from build123d import *

# Parameters (mm, degrees)
SKETCH_1_R               = 2
SKETCH_1_R_2             = 10
EXTRUDE_1_DEPTH          = 20
SKETCH_2_R               = 25
SKETCH_2_R_2             = 12
EXTRUDE_2_DEPTH          = 2
EXTRUDE_3_DEPTH          = 110
SKETCH_4_OUTSIDE_W       = 274.729
SKETCH_4_OUTSIDE_H       = 190.272
CUT_EXTRUDE_5_DEPTH      = 62
CUT_EXTRUDE_5_DEPTH_BACK = 62
SKETCH_5_R               = 7.5
EXTRUDE_4_DEPTH          = 55
SKETCH_6_R               = 5
EXTRUDE_5_DEPTH          = 40


with BuildPart() as part:
    # Эскиз1 → Бобышка-Вытянуть1 (new body)
    with BuildSketch(Plane(origin=(0, 0, 0), x_dir=(1, 0, 0), z_dir=(0, 1, 0))):
        with BuildLine():
            Line((35, 12.5), (35, -37))
            ThreePointArc((35, -37), (28.263455967, -53.263455967), (12, -60))
            Line((12, -60), (11, -60))
            Line((11, -60), (11, -67))
            ThreePointArc((11, -67), (10.121320344, -69.121320344), (8, -70))
            Line((8, -70), (-8, -70))
            ThreePointArc((-8, -70), (-10.121320344, -69.121320344), (-11, -67))
            Line((-11, -67), (-11, -60))
            Line((-11, -60), (-12, -60))
            ThreePointArc((-12, -60), (-28.263455967, -53.263455967), (-35, -37))
            Line((-35, -37), (-35, -35))
            Line((-35, -35), (-37, -35))
            ThreePointArc((-37, -35), (-39.121320344, -34.121320344), (-40, -32))
            Line((-40, -32), (-40, 12.5))
            ThreePointArc((-40, 12.5), (-40.878679656, 14.621320344), (-43, 15.5))
            Line((-43, 15.5), (-49, 15.5))
            ThreePointArc((-49, 15.5), (-57.485281374, 19.014718626), (-61, 27.5))
            Line((-61, 27.5), (-61, 28))
            ThreePointArc((-61, 28), (-57.485281374, 36.485281374), (-49, 40))
            Line((-49, 40), (49, 40))
            ThreePointArc((49, 40), (57.485281374, 36.485281374), (61, 28))
            Line((61, 28), (61, 27.5))
            ThreePointArc((61, 27.5), (57.485281374, 19.014718626), (49, 15.5))
            Line((49, 15.5), (38, 15.5))
            ThreePointArc((38, 15.5), (35.878679656, 14.621320344), (35, 12.5))
        make_face()
        with Locations((27.5, 27.5)):
            Circle(SKETCH_1_R, mode=Mode.SUBTRACT)
        with Locations((-27.5, 27.5)):
            Circle(SKETCH_1_R, mode=Mode.SUBTRACT)
        with Locations((-27.5, -27.5)):
            Circle(SKETCH_1_R, mode=Mode.SUBTRACT)
        with Locations((27.5, -27.5)):
            Circle(SKETCH_1_R, mode=Mode.SUBTRACT)
        Circle(SKETCH_1_R_2, mode=Mode.SUBTRACT)
    extrude(amount=EXTRUDE_1_DEPTH)

    # Эскиз2 → Бобышка-Вытянуть2 (add)
    with BuildSketch(Plane.XZ):
        Circle(SKETCH_2_R)
        Circle(SKETCH_2_R_2, mode=Mode.SUBTRACT)
    extrude(amount=EXTRUDE_2_DEPTH)

    # Эскиз3 → Бобышка-Вытянуть3 (add)
    with BuildSketch(Plane(origin=(0, 20, 0), x_dir=(1, 0, 0), z_dir=(0, 1, 0))):
        with BuildLine():
            Line((-37.583733624, -32.103535028), (-37.583733624, 36.457416544))
            Line((-37.583733624, 36.457416544), (-16, 36.457416544))
            Line((-16, 36.457416544), (-16, 146.457416544))
            Line((-16, 146.457416544), (16, 146.457416544))
            Line((16, 146.457416544), (16, 36.457416544))
            Line((16, 36.457416544), (33.766635678, 36.457416544))
            Line((33.766635678, 36.457416544), (33.766635678, -32.103535028))
            ThreePointArc((33.766635678, -32.103535028), (28.080470389, -50.220903637), (11.304482379, -59.11684357))
            Line((11.304482379, -59.11684357), (-11, -59.11684357))
            ThreePointArc((-11, -59.11684357), (-27.23731375, -51.101673534), (-33.326201299, -34.048264581))
            Line((-33.326201299, -34.048264581), (-37.583733624, -32.103535028))
        make_face()
    extrude(amount=EXTRUDE_3_DEPTH)

    # Эскиз4 outside → Вырез-Вытянуть5 (cut, two sides)
    with BuildSketch(Plane(origin=(0, 0, 0), x_dir=(0, 0, -1), z_dir=(1, 0, 0))) as cut_extrude_5_sk:
        with Locations((38.2285, 64)):
            Rectangle(SKETCH_4_OUTSIDE_W, SKETCH_4_OUTSIDE_H)
        Polygon((-59.11684357, 111.009140669), (-59.11684357, 20), (-70, 20), (-70, 0), (-25.61704501, 0), (-25.61704501, -2.465693048), (25.5, -2.465693048), (25.5, 0), (40, 0), (40, 20), (36.457416544, 20), (36.457416544, 70.826498743), (84.412407161, 70.826498743), (128.193178806, 61.67378586), (131.933723793, 56.499947934), (146.457416544, 56.499947934), (146.457416544, 83.32776512), (75.121913518, 98.241010205), (43.39244845, 98.241010205), (36.457416544, 102.079664685), (36.457416544, 126.416047598), (31.26241492, 130), (-26.036858243, 130), align=None, mode=Mode.SUBTRACT)
    extrude(amount=CUT_EXTRUDE_5_DEPTH, mode=Mode.SUBTRACT)
    extrude(cut_extrude_5_sk.sketch, amount=-CUT_EXTRUDE_5_DEPTH_BACK, mode=Mode.SUBTRACT)

    # Эскиз5 → Бобышка-Вытянуть4 (add)
    with BuildSketch(Plane.XZ.offset(-20)):
        Circle(SKETCH_5_R)
    extrude(amount=EXTRUDE_4_DEPTH)

    # Эскиз6 → Бобышка-Вытянуть5 (add)
    with BuildSketch(Plane.XZ.offset(35)):
        Circle(SKETCH_6_R)
    extrude(amount=EXTRUDE_5_DEPTH)


solid = part.part
CAD build for the part. Positions are in the model's coordinates, mm. A direction names the side the tool comes from. Coordinates: 2 decimals unless noted, no trailing zeros. Order: outer loops, then holes, each group sorted by start corner. A loop starts at its lowest first (then second) coordinate and runs counter-clockwise, first axis right, second up. Notation, with made-up numbers: (59.25, 52.25) -> (94.25, 52.25) arc R19 ccw to (94.25, 70.25) -> close; hole circle Ø10 at (50, 70.5). An arc over 180 degrees is marked (long way). Answer in a Markdown table with one row per item.
1) Drill centre lines: line 1 (Z direction, x = 0, y = 10.5); line 2 (Z direction, x = 27.5, y = 10.5); line 3 (Y direction, x = 52.5, z = -33). Where is each one in solid material? Low to high.
Check values:
| item | result |
|---|---|
| line 1 | -40 to -10, -7.5 to 7.5, 10 to 70 |
| line 2 | -40 to -29.5, -25.5 to 25.5, 29.5 to 53.99 |
| line 3 | 0 to 20 |
2) Mould opens along X. For faces 5 (the face through (-27.063, 71.963, 51.295)), 6 (the face through (0, 98.241, -59)), 7 (the face through (-2.17, 9.86, 9.76)) say: pulls with the +X half, pulls with the -X half, needs draft (parallel to the pull), parting line crosses it, or undercut.
Check values:
| item | result |
|---|---|
| face 5 | pulls with the -X half |
| face 6 | needs draft |
| face 7 | undercut |
3) Band-saw the part on A-A (y = 44). List the corners of the cut face in (x, z).
Check values:
| item | result |
|---|---|
| outline | (-37.58, -36.46) -> (33.77, -36.46) -> (33.77, 32.1) arc R25 ccw to (11.3, 59.12) -> (-11, 59.12) arc R24.13 ccw to (-33.33, 34.05) -> (-37.58, 32.1) -> close |
4) Band-saw the part on D-D (z = 22). List the corners of the cut face in (x, y), and give its area (3 significant figures).
Check values:
| item | result |
|---|---|
| outline | (-40, 0) -> (-11.87, 0) -> (-11.87, -2) -> (11.87, -2) -> (11.87, 0) -> (35, 0) -> (35, 20) -> (33.77, 20) -> (33.77, 130) -> (-37.58, 130) -> (-37.58, 20) -> (-40, 20) -> close |
| area | 9,400 mm2 |
5) Flat gauge pins, fed straight in: P1, Ø3, axis at x = 27.5, z = -27.5, coming from the -Y side; P2, Ø6, axis at y = 5.5, z = 11, coming from the +X side; P3, Ø0.8, axis at x = -11.5, y = 9.5, coming from the +Z side; P4, Ø4.5, axis at x = 27.5, z = 27.5, coming from the +Y side. Where does each tip first touch, or does it go through?
Check values:
| item | result |
|---|---|
| P1 | y = 20 |
| P2 | x = 35 |
| P3 | z = 60 |
| P4 | y = 130 |
6) Band-saw the part on C-C (y = 115.5). List the corners of the cut face in (x, z).
Check values:
| item | result |
|---|---|
| outline | (-37.58, -36.46) -> (33.77, -36.46) -> (33.77, 32.1) arc R25 ccw to (27.13, 51.29) -> (-27.06, 51.29) arc R24.13 ccw to (-33.33, 34.05) -> (-37.58, 32.1) -> close |
7) Band-saw the part on B-B (z = 0). List the corners of the cut face in (x, y).
Check values:
| item | result |
|---|---|
| outline | (-40, 0) -> (-25, 0) -> (-25, -2) -> (-12, -2) -> (-12, 0) -> (-10, 0) -> (-10, 20) -> (-7.5, 20) -> (-7.5, -35) -> (-5, -35) -> (-5, -75) -> (5, -75) -> (5, -35) -> (7.5, -35) -> (7.5, 20) -> (10, 20) -> (10, 0) -> (12, 0) -> (12, -2) -> (25, -2) -> (25, 0) -> (35, 0) -> (35, 20) -> (33.77, 20) -> (33.77, 130) -> (-37.58, 130) -> (-37.58, 20) -> (-40, 20) -> close |
8) Which spindle directions (+Z, -Z, +X, -X, +Y, -Y) get a long thin tool onto all of the face, cutting with end or side? Do faces 1 (the face through (-37.584, 74, -2)), 2 (the face through (-57.58, 9.86, -36.39)), 3 (the face through (0, 56.5, -139)), 4 (the face through (-4, 20, -7)). Say none if no direction does.
Check values:
| item | result |
|---|---|
| face 1 | +Z, -Z, -X, +Y |
| face 2 | -Z, -X, +Y, -Y |
| face 3 | -Z, +X, -X, -Y |
| face 4 | -Y |
